Build history of the part. All positions in model axes, mm. Round coordinates to 2 decimals unless told otherwise and drop trailing zeros. Order: outer loops, then holes, each group sorted by start corner. A loop starts at its lowest first (then second) coordinate and runs counter-clockwise, first axis right, second up. Notation, with made-up numbers: (-16, 11) -> (-11, 11) arc R27 cw to (-11, 45) -> close; hole circle Ø8 at (-11, -12). An arc over 180 degrees is marked (long way). Answer as a JSON object with one key per item and string values.
from build123d import *

# Parameters (mm, degrees)
SKETCH1_W         = 9.53
SKETCH1_H         = 9.53
BASIC_SHAPE_DEPTH = 4.83
SKETCH5_R         = 0.25
PINS_DEPTH        = 5
SKETCH6_W         = 0.5
SKETCH6_H         = 7.53
REAR_RELIEF_DEPTH = 19.035262682


with BuildPart() as part:
    # Sketch1 → Basic Shape (new body)
    with BuildSketch(Plane(origin=(0, 0, 0), x_dir=(0, 0, 1), z_dir=(1, 0, 0))):
        with Locations((4.765, 4.765)):
            Rectangle(SKETCH1_W, SKETCH1_H)
    extrude(amount=BASIC_SHAPE_DEPTH)

    # Sketch5 → Pins (add)
    with BuildSketch(Plane(origin=(0, -19.06, 0), x_dir=(0, -1, 0), z_dir=(0, 0, -1))):
        with Locations(Location((-16.835, -2.39, 0), (0, 0, 90))):
            Circle(SKETCH5_R)
        with Locations(Location((-14.295, -2.39, 0), (0, 0, 90))):
            Circle(SKETCH5_R)
        with Locations(Location((-11.755, -2.39, 0), (0, 0, 90))):
            Circle(SKETCH5_R)
    extrude(amount=PINS_DEPTH)

    # Sketch6 → Rear Relief (cut, through all)
    with BuildSketch(Plane.XY.offset(9.53)):
        with Locations((4.58, -4.765)):
            Rectangle(SKETCH6_W, SKETCH6_H)
    extrude(amount=-REAR_RELIEF_DEPTH, mode=Mode.SUBTRACT)


solid = part.part
1) Cut at A-A, the plane z = 1. Give the cut face in (x, y), plus the area to 3 significant figures.
Checked values:
{"outline": "(0, -9.53) -> (4.83, -9.53) -> (4.83, -8.53) -> (4.33, -8.53) -> (4.33, -1) -> (4.83, -1) -> (4.83, 0) -> (0, 0) -> close", "area": "42.3 mm²"}
2) Cut at C-C, the plane y = -6. Give the cut face in (x, z), plus the area to 3 significant figures.
Checked values:
{"outline": "(0, 0) -> (4.33, 0) -> (4.33, 9.53) -> (0, 9.53) -> close", "area": "41.3 mm²"}
3) Pull direction Y, two halves, no side cores. Call faces 1 (the face through (2, 0, 5)), 2 (the face through (2, -9.53, 5)), 3 (the face through (2, -5, 9.53)), 4 (the face through (4.33, -5, 5)): pulls with the +Y half, pulls with the -Y half, needs draft (parallel to the pull), parting line crosses it, or undercut.
Checked values:
{"face 1": "pulls with the +Y half", "face 2": "pulls with the -Y half", "face 3": "needs draft", "face 4": "undercut"}
4) Probe L1, parallel to Y at x = 4.4, z = 2.75; L2, parallel to X at y = -2.25, z = 5.75; L3, parallel to Z at x = 2.8, y = -3.5. List the from-to ranges inside material, lowest first. Write a range as from..to.
Checked values:
{"L1": "y = -9.53..-8.53, -1..0", "L2": "x = 0..4.33", "L3": "z = 0..9.53"}
5) Cut at D-D, the plane z = -3.5. Give the cut face in (x, y) (3 decimals).
Checked values:
{"outline": "circle Ø0.5 at (2.39, -7.305); circle Ø0.5 at (2.39, -4.765); circle Ø0.5 at (2.39, -2.225)"}
6) Cut at B-B, the plane x = 2.39. Give the cut face in (y, z) (3 decimals), plus the area to 3 significant figures.
Checked values:
{"outline": "(-9.53, 0) -> (-7.555, 0) -> (-7.555, -5) -> (-7.055, -5) -> (-7.055, 0) -> (-5.015, 0) -> (-5.015, -5) -> (-4.515, -5) -> (-4.515, 0) -> (-2.475, 0) -> (-2.475, -5) -> (-1.975, -5) -> (-1.975, 0) -> (0, 0) -> (0, 9.53) -> (-9.53, 9.53) -> close", "area": "98.3 mm²"}
